from build123d import *

# Parameters (mm, degrees)
BOSS_EXTRU_1_DEPTH            = 5
TROU_DE_PASSAGE_D_AXE_3_322_D = 2


with BuildPart() as part:
    # Esquisse1 → Boss.-Extru.1 (new body)
    with BuildSketch(Plane.XY):
        with BuildLine():
            Line((0, 14), (0, 0))
            Line((0, 0), (8.096774194, 0))
            ThreePointArc((8.096774194, 0), (15.096774194, 7), (8.096774194, 14))
            Line((8.096774194, 14), (0, 14))
        make_face()
    extrude(amount=BOSS_EXTRU_1_DEPTH)

    # Trou de passage d'axe 3/322 (through all)
    with Locations(Plane(origin=(7, 7, 5), x_dir=(1, 0, 0), z_dir=(0, 0, 1))):
        with Locations((0, 0)):
            Hole(TROU_DE_PASSAGE_D_AXE_3_322_D / 2)


solid = part.part
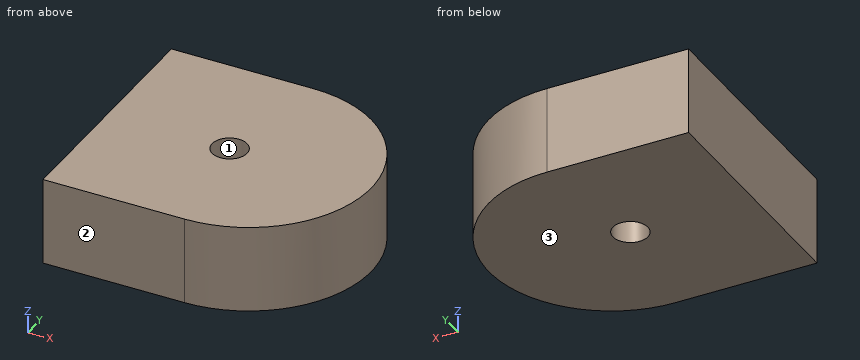
Model file for the job. Use its own axes, mm. Face numbers are marked on the shaded views. Give positions to 0.01 mm unless a question says otherwise; leave off trailing zeros. Loops run counter-clockwise (first coordinate to the right, second up) from the corner with the lowest first, then second, coordinate; pieces in that order, holes last.
Item 1: Slice it at C-C (y = 13). Write the cut outline in (x, z), plus the area to 3 significant figures.
Check values:
outline: (0, 0) - (11.7, 0) - (11.7, 5) - (0, 5) - close
area: 58.5 mm2
Item 2: Slice it at A-A (x = 7). Write the cut outline in (y, z), plus the area to 3 significant figures.
Check values:
outline: (0, 0) - (6, 0) - (6, 5) - (0, 5) - close; (8, 0) - (14, 0) - (14, 5) - (8, 5) - close
area: 60.0 mm2
Item 3: Drop a flat-ended pin along its axis: P1, Ø3, axis at x = 3, z = 2.5, coming from the -Y side. Give the stop position or say it passes through.
Check values:
P1: stops at y = 0
Item 4: Slice it at D-D (x = 13). Write the cut outline in (y, z), plus the area to 3 significant figures.
Check values:
outline: (2, 0) - (12, 0) - (12, 5) - (2, 5) - close
area: 50.0 mm2
Item 5: Drill centre lines: line 1 along Y through (x, z) = (7, 2); line 2 along X through (y, z) = (7.75, 3.4); line 3 along X through (y, z) = (11.75, 2.45). Where is each one in solid material? Low to high.
Check values:
line 1: y = 0 to 6, 8 to 14
line 2: x = 0 to 6.34, 7.66 to 15.06
line 3: x = 0 to 13.24
Item 6: Slice it at B-B (z = 4.05). Write the cut outline in (x, y), plus the area to 3 significant figures.
Check values:
outline: (0, 0) - (8.1, 0) arc R7 ccw to (8.1, 14) - (0, 14) - close; hole circle Ø2 at (7, 7)
area: 187 mm2
Item 7: Mould opens along Y. For the marked faces 1, 2 and 3 say: +Y half, -Y half, draft (parallel to the pull), parting line (faces both ways), or undercut.
Check values:
face 1: undercut
face 2: -Y half
face 3: draft
